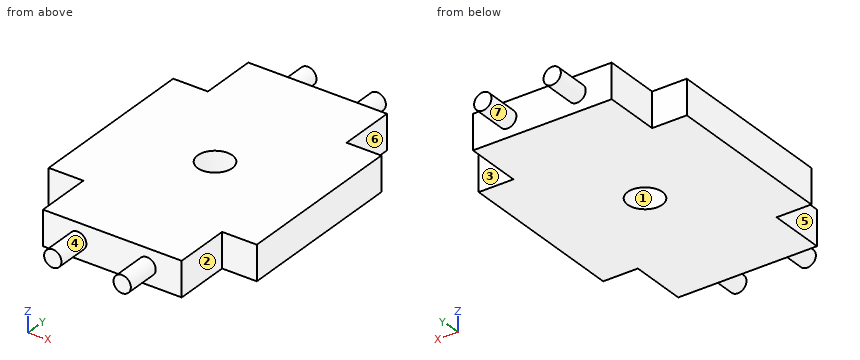
```python
from build123d import *

# Parameters (mm, degrees)
F0_R     = 3.175
F1_DEPTH = 6.35
F2_R     = 1.5875
F3_DEPTH = 6.35
F4_DEPTH = 6.35
F5_R     = 1.5875
F6_DEPTH = 6.35
F7_DEPTH = 6.35


with BuildPart() as f1:
    # F0 (on Top) → F1 (new body)
    with BuildSketch(Plane.XY):
        Polygon((12.7, 15.875), (12.7, 26.1747), (-12.7, 26.1747), (-12.7, 15.875), (-19.05, 15.875), (-19.05, -15.875), (-12.7, -15.875), (-12.7, -26.1747), (12.7, -26.1747), (12.7, -15.875), (19.05, -15.875), (19.05, 15.875), align=None)
        Circle(F0_R, mode=Mode.SUBTRACT)
    extrude(amount=F1_DEPTH)

    # F2 (on face) → F3 (join)
    with BuildSketch(Plane(origin=(0, 26.1747, 0), x_dir=(-1, 0, 0), z_dir=(0, 1, 0))):
        with Locations((-6.35, 3.175)):
            Circle(F2_R)
    extrude(amount=F3_DEPTH)

    # F2 (on face) → F4 (join)
    with BuildSketch(Plane(origin=(0, 26.1747, 0), x_dir=(-1, 0, 0), z_dir=(0, 1, 0))):
        with Locations((6.35, 3.175)):
            Circle(F2_R)
    extrude(amount=F4_DEPTH)

    # F5 (on face) → F6 (join)
    with BuildSketch(Plane.XZ.offset(26.1747)):
        with Locations((-6.35, 3.175)):
            Circle(F5_R)
    extrude(amount=F6_DEPTH)

    # F5 (on face) → F7 (join)
    with BuildSketch(Plane.XZ.offset(26.1747)):
        with Locations((-6.35, 3.175)):
            Circle(F5_R)
        with Locations((6.35, 3.175)):
            Circle(F5_R)
    extrude(amount=F7_DEPTH)


solid = f1.part
```
Check sheet for the modelled part. Datum: model origin and axes. Units: mm. Face numbers are marked on the shaded views. A direction names the side the tool comes from. Coordinates: 2 decimals unless noted, no trailing zeros. Write each loop counter-clockwise with the first axis right and the second up, starting at its lowest first coordinate (ties: lowest second). Pieces come first, ordered by that corner, then holes. Notation, with made-up numbers: M 41,-33.5 L 54,-33.5 A19 ccw 54,1.5 Z; hole C 13,84.5 d2. An arc over 180 degrees is marked long. Write item = value, one per line. Start each with the question number.
1. Mould release check, pull along Y, two halves, no side actions. Record for the marked faces 1, 2 and 3: pulls with the +Y half, pulls with the -Y half, needs draft (parallel to the pull), parting line crosses it, or undercut.
2. Tool access check on the marked faces 4, 5, 6 and 7. Record the directions out of +Z, -Z, +X, -X, +Y, -Y that give a thin tool (end or side, any length) a straight path to the whole face; none if there is none.
3. Sectioned sample at A-A (x = 0). Record the cut outline in (y, z) (3 decimals), then the cut area to 3 significant figures.
4. Thickness scan on probe 1 along Y at (x, z) = (0, 3.5) (3 decimals); probe 2 along Y at (x, z) = (-5.5, 1.5); probe 3 along X at (y, z) = (-23, 4.75). Record the ranges inside material, lowest first.
5. Sectioned sample at D-D (y = 22). Record the cut outline in (x, z), then the cut area to 3 significant figures.
6. Go/stop test with flat-tipped pins: pin 1 (1.9 mm diameter, centred on y = 22, z = 3, fed in from -X); pin 2 (1.9 mm diameter, centred on x = -16.5, z = 3, fed in from -Y) (3 decimals); pin 3 (2 mm diameter, centred on x = -12, z = 1, fed in from +Y); pin 4 (3 mm diameter, centred on y = 16.5, z = 4, fed in from +X). Record where each tip stops, or that it passes through.
7. Sectioned sample at C-C (x = -6.35). Record the cut outline in (y, z).
8. Sectioned sample at B-B (y = 0). Record the cut outline in (x, z) (3 decimals).
The answers:
q1.face_1 = undercut
q1.face_2 = needs draft
q1.face_3 = pulls with the +Y half
q2.face_4 = -Y
q2.face_5 = +Z, -Z, -X, -Y
q2.face_6 = +Z, -Z, +X, +Y
q2.face_7 = +Y
q3.outline = M -26.175,0 L -3.175,0 L -3.175,6.35 L -26.175,6.35 Z; M 3.175,0 L 26.175,0 L 26.175,6.35 L 3.175,6.35 Z
q3.area = 292 mm²
q4.probe_1 = -26.175 to -3.175, 3.175 to 26.175
q4.probe_2 = -26.17 to 26.17
q4.probe_3 = -12.7 to 12.7
q5.outline = M -12.7,0 L 12.7,0 L 12.7,6.35 L -12.7,6.35 Z
q5.area = 161 mm²
q6.pin_1 = -12.7
q6.pin_2 = -15.875
q6.pin_3 = 26.17
q6.pin_4 = 19.05
q7.outline = M -32.52,1.59 L -26.17,1.59 L -26.17,0 L 26.17,0 L 26.17,1.59 L 32.52,1.59 L 32.52,4.76 L 26.17,4.76 L 26.17,6.35 L -26.17,6.35 L -26.17,4.76 L -32.52,4.76 Z
q8.outline = M -19.05,0 L -3.175,0 L -3.175,6.35 L -19.05,6.35 Z; M 3.175,0 L 19.05,0 L 19.05,6.35 L 3.175,6.35 Z
